Geometry: final body of the model. Coordinates: model frame, mm. Face numbers are marked on the shaded views. A direction names the side the tool comes from. Give positions to 0.01 mm unless a question says otherwise; leave off trailing zeros. Write each loop counter-clockwise with the first axis right and the second up, starting at its lowest first coordinate (ties: lowest second). Pieces come first, ordered by that corner, then holes. Notation, with made-up numbers: M 18.25,-40 L 42.25,-40 A29 ccw 42.25,-6 Z; hole C -24.5,-3.75 d5. An arc over 180 degrees is marked long. Answer as a JSON object with one key per item and string values.
from build123d import *

# Parameters (mm, degrees)
CYLINDER_R     = 1.75
CYLINDER_DEPTH = 30
BOX001_W       = 20
BOX001_H       = 6
BOX001_DEPTH   = 3
PRISM_DEPTH    = 3


with BuildPart() as cilindro:
    # Cylinder → Cylinder (new body)
    with BuildSketch(Plane.XY.offset(-5)):
        Circle(CYLINDER_R)
    extrude(amount=CYLINDER_DEPTH)


with BuildPart() as cubo001:
    # Box001 → Box001 (new body)
    with BuildSketch(Plane(origin=(1, -3, 0), x_dir=(1, 0, 0), z_dir=(0, 0, 1))):
        with Locations((10, 3)):
            Rectangle(BOX001_W, BOX001_H)
    extrude(amount=BOX001_DEPTH)


with BuildPart() as fusion:
    # Prism → Prism (new body)
    with BuildSketch(Plane.XY):
        Polygon((3.25, 0), (1.625, 2.814583), (-1.625, 2.814583), (-3.25, 0), (-1.625, -2.814583), (1.625, -2.814583), align=None)
    extrude(amount=PRISM_DEPTH)

    # Fusion: union Cilindro, Cubo001
    add(cilindro.part)
    add(cubo001.part)


solid = fusion.part
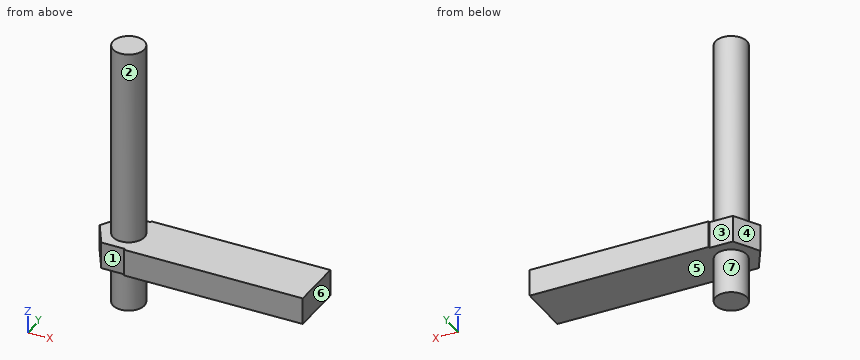
1) Cut plane B-B on y = -0.8. Return loops of the section in (x, z).
Geometry check:
{"outline": "M -2.79,0 L -1.56,0 L -1.56,-5 L 1.56,-5 L 1.56,0 L 21,0 L 21,3 L 1.56,3 L 1.56,25 L -1.56,25 L -1.56,3 L -2.79,3 Z"}
2) Contact query for flat-ended pins moving along their axis: P1, Ø2, axis at x = 16, y = 1, coming from the -Z side; P2, Ø2, axis at x = -1, z = 1, coming from the +Y side; P3, Ø12, axis at x = 17, z = 6, coming from the +Y side; P4, Ø0.8, axis at x = -0.5, z = 1.5, coming from the -Y side. Output: stop coordinate, or through.
Geometry check:
{"P1": "stops at z = 0", "P2": "stops at y = 2.81", "P3": "stops at y = 3", "P4": "stops at y = -2.81"}
3) Set-up query: the marked faces 1, 2 and 3. Return all of +Z, -Z, +X, -X, +Y, -Y with unobstructed straight access to the full face (end or side cutting, diameter ignored); none if empty.
Geometry check:
{"face 1": "+Z, -Z, -X, -Y", "face 2": "+Z", "face 3": "+Z, -Z, -X, +Y"}
4) Cut plane C-C on z = 11.25. Return loops of the section in (x, y), and give its area (3 significant figures).
Geometry check:
{"outline": "C 0,0 d3.5", "area": "9.62 mm2"}
5) Pull-direction query (X, two-part tool) for the marked faces 4, 5, 6 and 7; classes: pulls with the +X half, pulls with the -X half, needs draft (parallel to the pull), parting line crosses it, or undercut.
Geometry check:
{"face 4": "pulls with the -X half", "face 5": "needs draft", "face 6": "pulls with the +X half", "face 7": "parting line crosses it"}
6) Line query: line 1 (Z direction, x = 9, y = -0.5); line 2 (X direction, y = 0.05, z = -3); line 3 (X direction, y = 2, z = 0.75). Output: solid intervals per line, ascending. Write a range as from..to.
Geometry check:
{"line 1": "z = 0..3", "line 2": "x = -1.75..1.75", "line 3": "x = -2.1..21"}
7) Cut plane A-A on x = 0. Return loops of the section in (y, z).
Geometry check:
{"outline": "M -2.81,0 L -1.75,0 L -1.75,-5 L 1.75,-5 L 1.75,0 L 2.81,0 L 2.81,3 L 1.75,3 L 1.75,25 L -1.75,25 L -1.75,3 L -2.81,3 Z"}
8) Cut plane D-D on x = 3.5. Return loops of the section in (y, z).
Geometry check:
{"outline": "M -3,0 L 3,0 L 3,3 L -3,3 Z"}
